Input: part model. Units: mm. Frame: model coordinates. Face numbers are marked on the shaded views. A direction names the side the tool comes from. Give positions to 0.01 mm unless a question says otherwise; leave off trailing zeros. Loops run counter-clockwise (first coordinate to the right, second up) from the corner with the lowest first, then second, coordinate; pieces in that order, holes last.
from build123d import *

# Parameters (mm, degrees)
SALIENTE_EXTRUIR1_DEPTH = 30
CORTAR_EXTRUIR1_DEPTH   = 10
CROQUIS4_R              = 1.75
CORTAR_EXTRUIR2_DEPTH   = 10


with BuildPart() as part:
    # Croquis1 → Saliente-Extruir1 (new body)
    with BuildSketch(Plane.XY):
        with BuildLine():
            Line((26.421334586, 0), (26.421334586, 8))
            Line((26.421334586, 8), (7.816864755, 8))
            ThreePointArc((7.816864755, 8), (-10.078665414, 18.5), (-27.974195582, 8))
            Line((-27.974195582, 8), (-46.558360995, 7.201596348))
            Line((-46.558360995, 7.201596348), (-46.558360995, -0.993642206))
            Line((-46.558360995, -0.993642206), (-23.429695336, 0))
            ThreePointArc((-23.429695336, 0), (-10.078665414, 11.5), (3.272364509, 0))
            Line((3.272364509, 0), (26.421334586, 0))
        make_face()
    extrude(amount=SALIENTE_EXTRUIR1_DEPTH)

    # Croquis3 → Cortar-Extruir1 (cut)
    with BuildSketch(Plane(origin=(0, 8, 0), x_dir=(1, 0, 0), z_dir=(0, 1, 0))):
        Polygon((26.421334586, -2.25), (26.421334586, -27.75), (7.816864755, -27.75), (7.816864755, -33.359079395), (34.243736359, -33.359079395), (34.243736359, 4.857090857), (7.816864755, 4.857090857), (7.816864755, -2.25), align=None)
    extrude(amount=-CORTAR_EXTRUIR1_DEPTH, mode=Mode.SUBTRACT)

    # Croquis4 → Cortar-Extruir2 (cut)
    with BuildSketch(Plane(origin=(-0.394595422, 9.184861036, 0), x_dir=(0.99907843, 0.04292191, 0), z_dir=(-0.04292191, 0.99907843, 0))):
        with Locations((-42.706347949, -26)):
            Circle(CROQUIS4_R)
        with Locations((-42.706347949, -4)):
            Circle(CROQUIS4_R)
    extrude(amount=-CORTAR_EXTRUIR2_DEPTH, mode=Mode.SUBTRACT)


solid = part.part
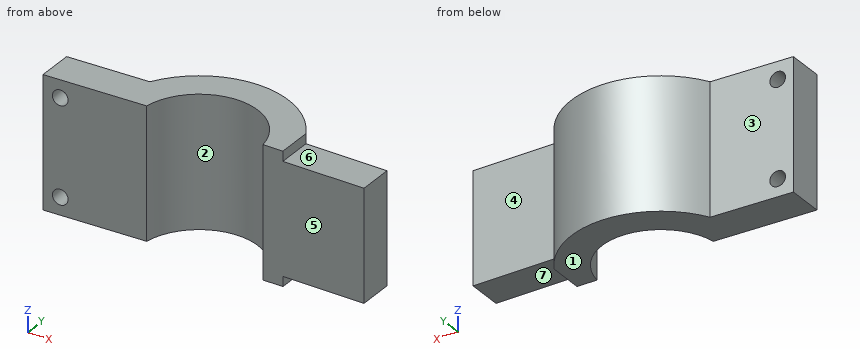
(1) Reachability of the marked faces 4, 5, 6 and 7 from +Z, -Z, +X, -X, +Y, -Y: full face, straight path, thin tool, end or side. Return the list, or none.
Values follow:
face 4: +Z, -Z, +X, +Y
face 5: +Z, -Z, +X, -Y
face 6: +Z, +X, +Y, -Y
face 7: -Z, +X, +Y, -Y
(2) Pin query (flat end, axial travel): pin 1 Ø1.1 at (y, z) = (2.5, 29.5) entering from +X; pin 2 Ø2 at (x, z) = (-32, 9) entering from +Y; pin 3 Ø7 at (x, z) = (10, 8.5) entering from -Y; pin 4 Ø2 at (x, y) = (1, 5) entering from +Z. Return the tip coordinate at first contact, or that it passes through.
Values follow:
pin 1: stops at x = 7.82
pin 2: stops at y = 7.87
pin 3: stops at y = 0
pin 4: stops at z = 30
(3) Ray query, probe 1 along Y at (x, z) = (14, 13); probe 2 along X at (y, z) = (4.5, 22.5); probe 3 along X at (y, z) = (6.75, 28.5). Return the intervals inside material, ascending.
Values follow:
probe 1: y = 0 to 8
probe 2: x = -46.56 to -21.91, 1.75 to 26.42
probe 3: x = -46.56 to -20.36, 0.2 to 7.82
(4) Cut plane B-B (z = 13.75). Return the cut outline in (x, y), and give its area (3 significant figures).
Values follow:
outline: (-46.56, -0.99) - (-23.43, 0) arc R13.5 cw to (3.27, 0) - (26.42, 0) - (26.42, 8) - (7.82, 8) arc R20.5 ccw to (-27.97, 8) - (-46.56, 7.2) - close
area: 622 mm2
(5) Cut plane A-A (y = 10.5). Return the cut outline in (x, z), and give its area (3 significant figures).
Values follow:
outline: (-26.33, 0) - (-15.18, 0) - (-15.18, 30) - (-26.33, 30) - close; (-4.98, 0) - (6.17, 0) - (6.17, 30) - (-4.98, 30) - close
area: 669 mm2
(6) Cut plane D-D (x = 21). Return the cut outline in (y, z), and give its area (3 significant figures).
Values follow:
outline: (0, 2.25) - (8, 2.25) - (8, 27.75) - (0, 27.75) - close
area: 204 mm2
(7) Cut plane C-C (y = 5). Count the separate pieces of the cut face and the enclosed holes in it, and give its area (3 significant figures).
Values follow:
separate pieces: 2
enclosed holes: 2
area: 1,390 mm2
(8) Mould query, pull axis X, two halves, no side actions, for the marked faces 1, 2 and 3. Classes: +X half, -X half, draft (parallel to the pull), parting line (faces both ways), or undercut.
Values follow:
face 1: draft
face 2: undercut
face 3: -X half
